from build123d import *

# Parameters (mm, degrees)
F2_R     = 5.08
F3_R     = 1.905
F3_W     = 7.62
F3_H     = 2.54
F4_DEPTH = 10.16


with BuildPart() as f1:
    # F0 (on Front) → F1 (revolve)
    with BuildSketch(Plane.XZ):
        Polygon((12.7, 50.8), (12.7, 0), (25.4, 0), (19.05, 31.75), (25.4, 50.8), align=None)
    revolve(axis=Axis((12.7, 0, 25.4), (0, 0, -1)))

    # F2
    f2_edges = [f1.edges().sort_by_distance(p)[0] for p in [
        (0, 0, 50.8),
    ]]
    fillet(f2_edges, radius=F2_R)

    # F3 (on Front) → F4 (join)
    with BuildSketch(Plane.XZ):
        with Locations((7.62, 40.3035629486)):
            Circle(F3_R)
        with Locations((17.78, 40.3035629486)):
            Circle(F3_R)
        with Locations((12.7, 36.4935629486)):
            Rectangle(F3_W, F3_H)
    extrude(amount=F4_DEPTH)


solid = f1.part
Can you work these out from the model? Positions are in its coordinate system, mm. A direction names the side the tool comes from. Coordinates: 2 decimals unless noted, no trailing zeros. Loops run counter-clockwise (first coordinate to the right, second up) from the corner with the lowest first, then second, coordinate; pieces in that order, holes last. Notation, with made-up numbers: M -19.75,36.5 L 13.25,36.5 A23 cw 13.25,72.5 Z; hole C 70.25,14.5 d11. An arc over 180 degrees is marked long. Return JSON: item names as keys, results as strings. Group by question number.
Item 1: Imagine slicing it at D-D (z = 13.5). Please give me the cut outline in (x, y), and give its area (3 significant figures).
Item 2: I'm going to push flat-ended pins straight in: pin 1 Ø6 at (x, z) = (18.5, 10) entering from +Y; pin 2 Ø2 at (y, z) = (3, 25.5) entering from +X; pin 3 Ø5 at (y, z) = (4, 28) entering from +X. Where does each tip first touch, or does it pass through?
Item 3: Imagine slicing it at C-C (x = 12.7). Please give me the cut outline in (y, z), and give its area (3 significant figures).
Item 4: Imagine slicing it at B-B (z = 24.5). Please give me the cut outline in (x, y).
Item 5: On a 3-axis mill with a long thin cutter (end or side, diameter ignored), from which of +Z, -Z, +X, -X, +Y, -Y can I reach the whole of each face in a straight line? I mean faces 1 (the flat face through (8.89, -9, 36)), 2 (the flat face through (16.51, -9, 36)), 3 (the conical face through (20.806, 3.361, 19.625)). Say none if no direction works.
Item 6: If I drill on L1, parallel to X at y = 5, z = 5.5; L2, parallel to Y at x = 9, z = 12; L3, parallel to Z at x = 15.5, y = 5.5, over which ranges is the centre line in solid material (lowest first)? Write a range as from..to.
Item 7: Imagine slicing it at A-A (y = 0). Please give me the cut outline in (x, z).
Item 8: Thinking about a two-plate mould opening in Z: for faces 4 (the flat face through (13, 0, 50.8)), 5 (the flat face through (13, 0, 0)), 6 (the flat face through (13, -10.16, 37)), which applies, released by +Z, released by -Z, zero draft, split by the parting line, or undercut?
Verdict:
{
 "1": {"outline": "C 12.7,0 d20", "area": "314 mm^2"},
 "2": {"pin 1": "stops at y = 10.53", "pin 2": "stops at x = 20.1", "pin 3": "stops at x = 19.82"},
 "3": {"outline": "M -12.7,0 L 12.7,0 L 6.35,31.75 L 10.47,44.11 A5.08 ccw 5.65,50.8 L -5.65,50.8 A5.08 ccw -10.47,44.11 L -8.35,37.76 L -10.16,37.76 L -10.16,35.22 L -7.51,35.22 L -6.35,31.75 Z", "area": "951 mm^2"},
 "4": {"outline": "C 12.7,0 d15.6"},
 "5": {"face 1": "-X, -Y", "face 2": "+X, -Y", "face 3": "none"},
 "6": {"L1": "x = 2.23..23.17", "L2": "y = -9.61..9.61", "L3": "z = 0..50.77"},
 "7": {"outline": "M 0,0 L 25.4,0 L 19.05,31.75 L 23.17,44.11 A5.08 ccw 18.35,50.8 L 7.05,50.8 A5.08 ccw 2.23,44.11 L 6.35,31.75 Z"},
 "8": {"face 4": "released by +Z", "face 5": "released by -Z", "face 6": "undercut"}
}
